Part model, mm, in its own coordinate system. Face numbers are marked on the shaded views. Give positions to 0.01 mm unless a question says otherwise; leave off trailing zeros. Loops run counter-clockwise (first coordinate to the right, second up) from the corner with the lowest first, then second, coordinate; pieces in that order, holes last. Notation, with made-up numbers: (21, 2.5) -> (78, 2.5) arc R15 cw to (78, 21.5) -> close; hole circle Ø7 at (56.25, 49). An arc over 180 degrees is marked (long way). Write item = value, one per line.
from build123d import *

# Parameters (mm, degrees)
F0_R     = 43.266566
F1_DEPTH = 12.7
F2_DEPTH = 63.5
F4_DEPTH = 50.8
F6_DEPTH = 80.962192


with BuildPart() as f1:
    # F0 (on Top) → F1 (new body)
    with BuildSketch(Plane.XY):
        with BuildLine():
            ThreePointArc((47.97375, -54.980806), (117.011051, -59.185378), (152.800973, 0))
            ThreePointArc((152.800973, 0), (117.011051, 59.185378), (47.97375, 54.980806))
            ThreePointArc((47.97375, 54.980806), (19.13688, 0), (47.97375, -54.980806))
        make_face()
        with Locations((85.968927, 0)):
            Circle(F0_R, mode=Mode.SUBTRACT)
        with BuildLine():
            ThreePointArc((47.97375, -54.980806), (19.13688, 0), (47.97375, 54.980806))
            Line((47.97375, 54.980806), (-113.462299, 54.980806))
            Line((-113.462299, 54.980806), (-113.462299, -54.980806))
            Line((-113.462299, -54.980806), (47.97375, -54.980806))
        make_face()
    extrude(amount=F1_DEPTH)

    # F0 (on Top) → F2 (join)
    with BuildSketch(Plane.XY):
        with BuildLine():
            ThreePointArc((47.97375, -54.980806), (117.011051, -59.185378), (152.800973, 0))
            ThreePointArc((152.800973, 0), (117.011051, 59.185378), (47.97375, 54.980806))
            ThreePointArc((47.97375, 54.980806), (19.13688, 0), (47.97375, -54.980806))
        make_face()
        with Locations((85.968927, 0)):
            Circle(F0_R, mode=Mode.SUBTRACT)
    extrude(amount=F2_DEPTH)

    # F3 (on face) → F4 (join)
    with BuildSketch(Plane.XY.offset(12.7)):
        with BuildLine():
            ThreePointArc((20.507041, -13.463432), (19.13688, 0), (20.507041, 13.463432))
            Line((20.507041, 13.463432), (-68.548821, 13.463432))
            Line((-68.548821, 13.463432), (-68.548821, -14.129145))
            Line((-68.548821, -14.129145), (20.507041, -14.129145))
            Line((20.507041, -14.129145), (20.507041, -13.463432))
        make_face()
    extrude(amount=F4_DEPTH)

    # F5 (on face) → F6 (cut, through all)
    with BuildSketch(Plane.XZ.offset(14.129145)):
        Polygon((-68.548821, 12.7), (20.507041, 63.5), (-68.548821, 63.5), align=None)
    extrude(amount=-F6_DEPTH, mode=Mode.SUBTRACT)


solid = f1.part
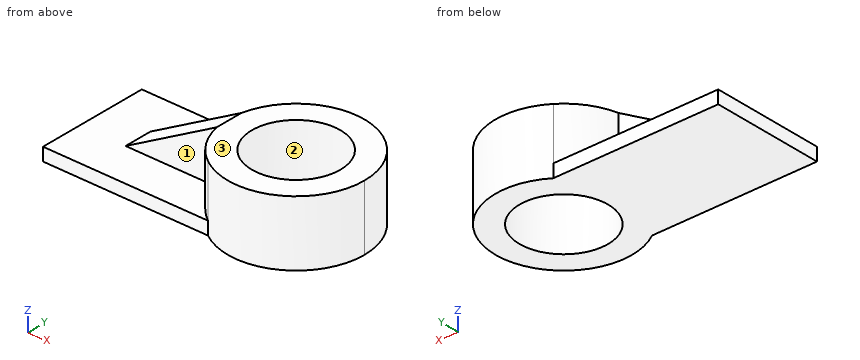
1) Slice it at C-C, the plane z = 24. List the corners of the cut face in (x, y).
Resolved:
outline = (-48.74, -14.13) -> (20.51, -14.13) -> (20.51, -13.46) arc R66.83 ccw (long way) to (20.51, 13.46) -> (-48.74, 13.46) -> close; hole circle Ø86.53 at (85.97, 0)
2) Drop flat-ended pins along their axis: P1, Ø3, axis at y = 45.5, z = 28.5, coming from the -X side; P2, Ø3, axis at y = -37, z = 34.5, coming from the -X side; P3, Ø8, axis at y = 52.5, z = 38, coming from the +X side. Give the stop position or say it passes through.
Resolved:
P1 = 35.66
P2 = 29.34
P3 = 131.95
3) Drill centre lines: line 1 along Z through (x, y) = (-29, 39); line 2 along Y through (x, z) = (-39, 3); line 3 along Y through (x, z) = (82.5, 59). Where is each one in solid material? Low to high. Write a range as [from, to].
Resolved:
line_1 = [0, 12.7]
line_2 = [-54.98, 54.98]
line_3 = [-66.74, -43.13], [43.13, 66.74]
4) Pull direction Y, two halves, no side cores. Call the marked faces 1, 2 and 3: pulls with the +Y half, pulls with the -Y half, needs draft (parallel to the pull), parting line crosses it, or undercut.
Resolved:
face_1 = pulls with the -Y half
face_2 = undercut
face_3 = needs draft
5) Slice it at D-D, the plane x = -19. List the corners of the cut face in (y, z), and give its area (3 significant figures).
Resolved:
outline = (-54.98, 0) -> (54.98, 0) -> (54.98, 12.7) -> (13.46, 12.7) -> (13.46, 40.96) -> (-14.13, 40.96) -> (-14.13, 12.7) -> (-54.98, 12.7) -> close
area = 2,180 mm²
6) Slice it at A-A, the plane y = -21.5. List the corners of the cut face in (x, z), and give its area (3 significant figures).
Resolved:
outline = (-113.46, 0) -> (48.42, 0) -> (48.42, 63.5) -> (22.69, 63.5) -> (22.69, 12.7) -> (-113.46, 12.7) -> close; (123.52, 0) -> (149.25, 0) -> (149.25, 63.5) -> (123.52, 63.5) -> close
area = 5,000 mm²
7) Slice it at B-B, the plane x = 99. List the corners of the cut face in (y, z), and give its area (3 significant figures).
Resolved:
outline = (-65.55, 0) -> (-41.26, 0) -> (-41.26, 63.5) -> (-65.55, 63.5) -> close; (41.26, 0) -> (65.55, 0) -> (65.55, 63.5) -> (41.26, 63.5) -> close
area = 3,090 mm²
